For this review, take the finished solid that the model builds, in its own axes (mm). A direction names the side the tool comes from. Coordinates: 2 decimals unless noted, no trailing zeros. Loops run counter-clockwise (first coordinate to the right, second up) from the corner with the lowest first, then second, coordinate; pieces in that order, holes last. Notation, with made-up numbers: M 20,87.25 L 25,87.25 A23 ccw 25,109.25 Z; hole C 50,-37 d11. An arc over 180 degrees is marked long. Write each question's results on one line, items separated by ' | '. Start each with the question number.
Autodesk Inventor part; units mm, degrees
ref_plane "YZ Plane" through (0, 0, 0) normal (1, 0, 0) x (0, 1, 0)
ref_plane "XZ Plane" through (0, 0, 0) normal (0, 1, 0) x (-1, 0, 0)
ref_plane "XY Plane" through (0, 0, 0) normal (0, 0, 1) x (1, 0, 0)
sketch "Sketch1" plane through (0, 0, 0) normal (1, 0, 0) x (0, 1, 0)
  line L0 (-9.5, 9.5) -> (9.5, 9.5)
  line L1 (9.5, 9.5) -> (9.5, -9.5)
  line L2 (9.5, -9.5) -> (-9.5, -9.5)
  line L3 (-9.5, -9.5) -> (-9.5, 9.5)
  line L4 (-9.5, 9.5) -> (9.5, -9.5) construction
  line L5 (9.5, 9.5) -> (-9.5, -9.5) construction
  line L6 (-7.5, 7.5) -> (7.5, 7.5)
  line L7 (7.5, 7.5) -> (7.5, -7.5)
  line L8 (7.5, -7.5) -> (-7.5, -7.5)
  line L9 (-7.5, -7.5) -> (-7.5, 7.5)
  line L10 (-7.5, 7.5) -> (7.5, -7.5) construction
  line L11 (7.5, 7.5) -> (-7.5, -7.5) construction
  point P0 (0, 0)
  dimension "d0" = 2
  dimension "d1" = 2
  dimension "d2" = 19
  dimension "d3" = 19
extrude "Extrusion1" add sketch "Sketch1" along normal blind 400
sketch "Sketch2" plane through (0, -9.5, 9.5) normal (0, 0, 1) x (1, 0, 0)
  line L0 (0, 19) -> (0, 0)
  line L1 (0, 19) -> (400, 19)
  line L2 (400, 19) -> (400, 0)
  line L3 (0, 0) -> (400, 0)
  line L4 (0, 0) -> (19, 19)
  line L5 (400, 0) -> (381, 19)
  point P0 (0, 9.5)
  dimension "d10" = 45
  dimension "d11" = 45
extrude "Extrusion2" cut sketch "Sketch2" against normal through all contours L1 L4 L0 | L5 L1 L2
equation "\"d1\" = d0"
properties part number "RS2_TubeFoot" material "Steel"
Q1. For faces 5 (the face through (197, -7.5, 0)), 6 (the face through (197, -9.5, 0)), list the 3-axis set-ups (+Z, -Z, +X, -X, +Y, -Y) from which the entire face can be reached by the end or side of a thin tool; tool diameter is ignored.
Q2. Take a section at B-B, the plane y = 1.75. Give the boundary of the cut face in (x, z).
Q3. Take a section at A-A, the plane z = 3.75. Give the boundary of the cut face in (x, y).
Q4. The part is to be moulded in two halves that separate along Z. For faces 1 (the face through (197, 0, -9.5)), 2 (the face through (9.4, -0.1, -8.3)), 3 (the face through (197, 0, 9.5)), 4 (the face through (197, 0, -7.5)), say which applies: pulls with the +Z half, pulls with the -Z half, needs draft (parallel to the pull), parting line crosses it, or undercut.
Q5. To check wall thickness, follow line 1 along Z through (x, y) = (23, 7); line 2 along X through (y, z) = (8.75, -3.5). State the ranges of each line that lie inside material, in increasing order.
Q6. Take a section at C-C, the plane x = 203. Give the boundary of the cut face in (y, z).
Results:
1) face 5: +X, -X | face 6: +Z, -Z, +X, -X, -Y
2) outline: M 11.25,-9.5 L 388.75,-9.5 L 388.75,-7.5 L 11.25,-7.5 Z; M 11.25,7.5 L 388.75,7.5 L 388.75,9.5 L 11.25,9.5 Z
3) outline: M 0,-9.5 L 400,-9.5 L 398,-7.5 L 2,-7.5 Z; M 17,7.5 L 383,7.5 L 381,9.5 L 19,9.5 Z
4) face 1: pulls with the -Z half | face 2: needs draft | face 3: pulls with the +Z half | face 4: undercut
5) line 1: -9.5 to -7.5, 7.5 to 9.5 | line 2: 18.25 to 381.75
6) outline: M -9.5,-9.5 L 9.5,-9.5 L 9.5,9.5 L -9.5,9.5 Z; hole M -7.5,-7.5 L 7.5,-7.5 L 7.5,7.5 L -7.5,7.5 Z
